Autodesk Inventor part; units mm, degrees
ref_plane "Work Plane1" through (4.77, 2.8444, 22.011) normal (0, 0, 1) x (1, 0, 0)
ref_plane "YZ Plane" through (0, 0, 0) normal (1, 0, 0) x (0, 1, 0)
ref_plane "XZ Plane" through (0, 0, 0) normal (0, 1, 0) x (-1, 0, 0)
ref_plane "Work Plane1" through (4.77, 2.8444, 22.011) normal (0, 0, 1) x (1, 0, 0)
sketch "Sketch1" plane through (0, 0, 0) normal (0, 0, 1) x (1, 0, 0)
  line L0 (0.5, -10) -> (-5.5, -10)
  line L1 (-5.5, -10) -> (-5.5, 10)
  line L2 (-5.5, 10) -> (0.5, 10)
  line L3 (0.5, 10) -> (0.5, -10)
  line L4 (-4, 8) -> (-4, -8) construction
  line L5 (0, 8) -> (-4, 8) construction
  line L6 (0, -8) -> (-4, -8) construction
  line L7 (0.5, -14.6916) -> (0.5, 15.0789) construction
  point P0 (0, 0)
  dimension "d0" = 2
  dimension "d1" = 2
  dimension "d3" = 6
  dimension "d4" = 0
extrude "Extrusion1" add sketch "Sketch1" along normal mid plane 60
sketch "Sketch2" plane through (0.5, -10, 30) normal (1, 0, 0) x (0, 0, -1)
  line L0 (47.5, 18) -> (12.5, 18)
  line L1 (12.5, 18) -> (12.5, 2)
  line L2 (12.5, 2) -> (47.5, 2)
  line L3 (47.5, 2) -> (47.5, 18)
  line L4 (41.725, 8.15) -> (18.275, 8.15)
  arc A0 (17.675, 8.75) -> (18.275, 8.15) centre (18.275, 8.75) ccw
  line L5 (17.675, 8.75) -> (17.675, 11.25)
  arc A1 (18.275, 11.85) -> (17.675, 11.25) centre (18.275, 11.25) ccw
  line L6 (18.275, 11.85) -> (41.725, 11.85)
  arc A2 (42.325, 11.25) -> (41.725, 11.85) centre (41.725, 11.25) ccw
  line L7 (42.325, 11.25) -> (42.325, 8.75)
  arc A3 (41.725, 8.15) -> (42.325, 8.75) centre (41.725, 8.75) ccw
  point P0 (30, 10)
extrude "Extrusion2" cut sketch "Sketch2" against normal blind 4 contours L3 L2 L1 L0 | L4 A0 L5 A1 L6 A2 L7 A3
sketch "Sketch3" plane through (0, 0, 30) normal (0, 0, 1) x (1, 0, 0)
  arc A0 (13.2615, 6.3791) -> (13.2616, 6.3779) centre (19.25, 6.75) ccw construction
  line L0 (-5.5, -10) -> (0.5, -10)
  line L1 (0.5, 10) -> (-5.5, 10)
  line L2 (0.5, 10) -> (0.5, -10)
  circle A1 centre (19.25, 6.75) radius 1.375
  line L3 (4.77, 6.75) -> (24.4771, 6.75) construction
  line L4 (24.25, 3.4334) -> (24.25, 10.0666)
  line L5 (22.5666, 11.75) -> (15.9334, 11.75)
  line L6 (24.25, 6.75) -> (19.25, 6.75) construction
  line L7 (19.25, 11.75) -> (19.25, 6.75) construction
  arc A2 (18.6093, 0.7843) -> (22.5666, 11.75) centre (19.25, 6.75) ccw
  line L8 (15.9334, 11.75) -> (0.5, 10)
  line L9 (0.5, -10) -> (24.25, 3.4334)
  arc A3 (2.5, 31.5) -> (-5.5, -10) centre (19.25, 6.75) ccw construction
  line L10 (0.5, -10) -> (0.5, 10) construction
  arc A4 (2.5, 25.5) -> (0.5, -10) centre (19.25, 6.75) ccw construction
  line L11 (2.5, 31.5) -> (2.5, 25.5) construction
  line L12 (2.77, 3.75) -> (0.5, 3.75) construction
  point P0 (0, 0)
  point P1 (19.25, 12.75)
  dimension "d12" = 2.75
  dimension "d13" = 6
  dimension "d18" = 1
  dimension "d19" = 2
  dimension "d20" = 3
extrude "Extrusion3" add sketch "Sketch3" against normal blind 3 contours L8 L5 A2 L4 L9 L2
mirror "Mirror1" about plane through (0, 0, 0) normal (0, 0, 1) of "Extrusion3"
Work out the finished part from the listing and answer in its coordinate system (mm). A direction names the side the tool comes from. Coordinates: 2 decimals unless noted, no trailing zeros. Order: outer loops, then holes, each group sorted by start corner. A loop starts at its lowest first (then second) coordinate and runs counter-clockwise, first axis right, second up. Notation, with made-up numbers: (71, -10) - (99, -10) arc R12 cw to (99, 0) - close; hole circle Ø11 at (57, -2). An arc over 180 degrees is marked (long way). Put each result on its own line as item: value. Start each with the question number.
1) Flat-ended cylindrical pins translate along their axes: pin 1 (2 mm diameter, centred on x = -2, z = -6, fed in from +Y); pin 2 (6 mm diameter, centred on y = 4, z = 11.5, fed in from +X). Find the tip coordinate at first contact, or state that the pin passes through.
2) Find section A-A (x = -0.5). Give the vertices of the cut face in (y, z), plus the area to 3 significant figures.
3) For a pull along Z with two mould halves and no side action, classify faces 4 (the flat face through (12.54, -3.19, -28.52)), 5 (the flat face through (0.5, -9, 0)), 6 (the flat face through (6, 3, 30)) as released by +Z, released by -Z, zero draft, split by the parting line, or undercut.
4) Find section C-C (z = -15). Give the vertices of the cut face in (x, y).
5) Find the intervals of material crossed by line 1 (Y direction, x = -0.5, z = -2); line 2 (Z direction, x = 16, y = -1); line 3 (X direction, y = 6, z = 14), in increasing order. Write a range as from..to.
6) For faces 1 (the flat face through (8.109, 10.863, -28.521)), 2 (the flat face through (10, 3, -27)), 3 (the flat face through (-1, 0, -17.5)), determine the directions among +Z, -Z, +X, -X, +Y, -Y from which every point of the face is accessible in a straight line to the end or side of a thin tool.
7) Find section B-B (y = 9.25). Give the vertices of the cut face in (x, z).
8) Find section D-D (x = 19.25). Give the vertices of the cut face in (y, z) (3 decimals), plus the area to 3 significant figures.
Results list:
1. pin 1: stops at y = 10
1. pin 2: stops at x = -3.5
2. outline: (-10, -30) - (10, -30) - (10, 30) - (-10, 30) - close; hole (-8, -17.5) - (8, -17.5) - (8, 17.5) - (-8, 17.5) - close
2. area: 640 mm^2
3. face 4: zero draft
3. face 5: undercut
3. face 6: released by +Z
4. outline: (-5.5, -10) - (0.5, -10) - (0.5, -8) - (-3.5, -8) - (-3.5, 8) - (0.5, 8) - (0.5, 10) - (-5.5, 10) - close
5. line 1: y = -10..-8, 8..10
5. line 2: z = -30..-27, 27..30
5. line 3: x = -5.5..-3.5
6. face 1: +Z, -Z, -X, +Y
6. face 2: +X, +Y, -Y
6. face 3: +X
7. outline: (-5.5, -30) - (24.25, -30) - (24.25, -27) - (0.5, -27) - (0.5, 27) - (24.25, 27) - (24.25, 30) - (-5.5, 30) - close
8. outline: (0.605, -30) - (5.375, -30) - (5.375, -27) - (0.605, -27) - close; (0.605, 27) - (5.375, 27) - (5.375, 30) - (0.605, 30) - close; (8.125, -30) - (11.75, -30) - (11.75, -27) - (8.125, -27) - close; (8.125, 27) - (11.75, 27) - (11.75, 30) - (8.125, 30) - close
8. area: 50.4 mm^2
